Answer from the drawing. Dimensions are ordinates in mm from the lowest x, y and z of the part. A direction names the side the tool comes from. Round coordinates to 2 decimals unless told otherwise and drop trailing zeros. Loops run counter-clockwise (first coordinate to the right, second up) from the corner with the lowest first, then second, coordinate; pieces in that order, holes last. Notation, with made-up numbers: M -3.75,59.25 L 9.25,59.25 A24 ccw 9.25,87.25 Z; hole C 3.25,14 d3. An arc over 180 degrees is marked long. One line per item, written item: value.
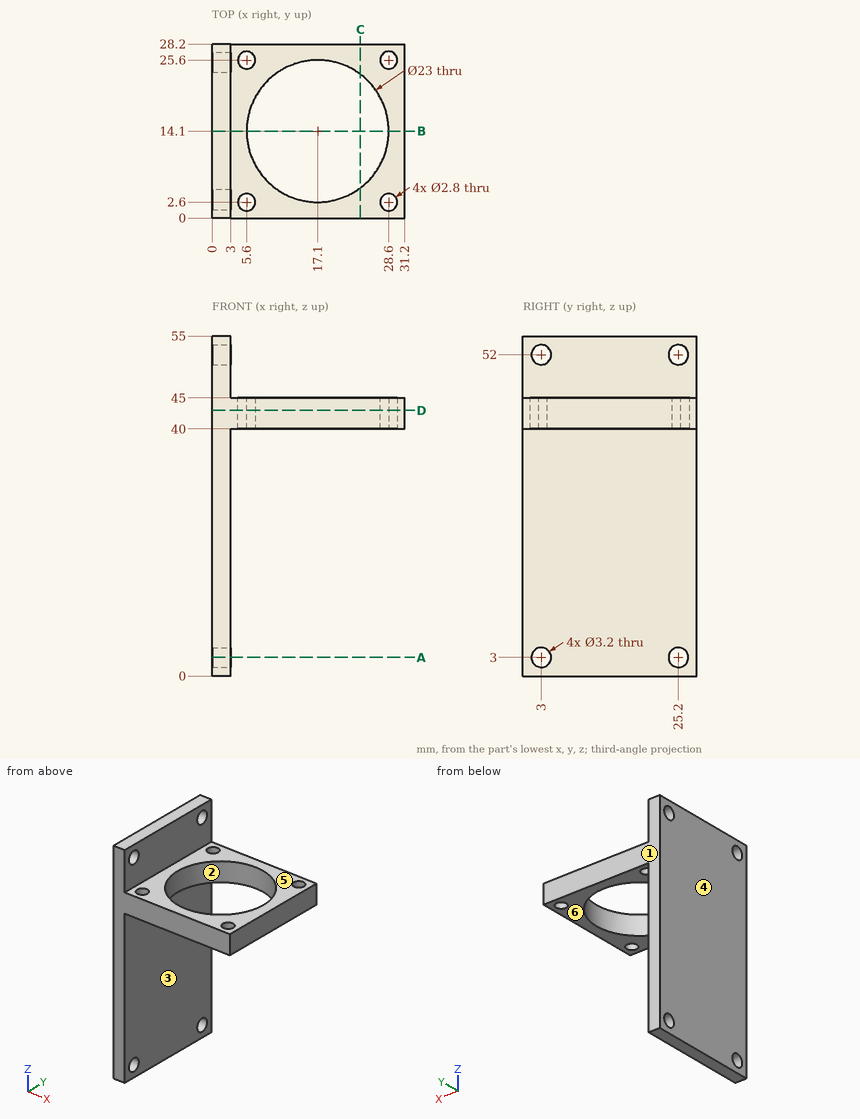
1) Find section C-C (x = 24). Give the vertices of the cut face in (y, z).
Check values:
outline: M 0,40 L 4.9,40 L 4.9,45 L 0,45 Z; M 23.3,40 L 28.2,40 L 28.2,45 L 23.3,45 Z
2) Find the intervals of material crossed by probe 1 along Z at (x, y) = (1.45, 25.2); probe 2 along X at (y, z) = (26.5, 24.5); probe 3 along Z at (x, y) = (29.5, 15.5), in increasing order. Write a range as from..to.
Check values:
probe 1: 0..1.4, 4.6..50.4, 53.6..55
probe 2: 0..3
probe 3: 40..45
3) Each of these flat-tipped pins is pushed along its axis until it touches: pin 1 (1.7 mm diameter, centred on x = 28.6, y = 25.6, fed in from +Z); pin 2 (3 mm diameter, centred on y = 11.5, z = 49, fed in from +X); pin 3 (4.5 mm diameter, centred on x = 5.6, y = 2.6, fed in from +Z); pin 4 (10 mm diameter, centred on x = 23, z = 46, fed in from +Y). Where does it stop, or does it pass through?
Check values:
pin 1: through
pin 2: x = 3
pin 3: z = 45
pin 4: y = 28.2
4) The mould has two halves that part along X. Classify the marked faces 1, 2 and 3: +X half, -X half, draft (parallel to the pull), parting line (faces both ways), or undercut.
Check values:
face 1: draft
face 2: undercut
face 3: +X half
5) Find section B-B (y = 14.1). Give the vertices of the cut face in (x, z).
Check values:
outline: M 0,0 L 3,0 L 3,40 L 5.6,40 L 5.6,45 L 3,45 L 3,55 L 0,55 Z; M 28.6,40 L 31.2,40 L 31.2,45 L 28.6,45 Z
6) For the marked faces 4, 5 and 6, determine the directions among +Z, -Z, +X, -X, +Y, -Y from which every point of the face is accessible in a straight line to the end or side of a thin tool.
Check values:
face 4: +Z, -Z, -X, +Y, -Y
face 5: +Z, +X, +Y, -Y
face 6: -Z, +X, +Y, -Y
7) Find section A-A (z = 3). Give the vertices of the cut face in (x, y).
Check values:
outline: M 0,0 L 3,0 L 3,1.4 L 0,1.4 Z; M 0,4.6 L 3,4.6 L 3,23.6 L 0,23.6 Z; M 0,26.8 L 3,26.8 L 3,28.2 L 0,28.2 Z
8) Find section D-D (z = 43). Give the vertices of the cut face in (x, y), then the cut area to 3 significant figures.
Check values:
outline: M 0,0 L 31.2,0 L 31.2,28.2 L 0,28.2 Z; hole C 5.6,2.6 d2.8; hole C 5.6,25.6 d2.8; hole C 17.1,14.1 d23; hole C 28.6,2.6 d2.8; hole C 28.6,25.6 d2.8
area: 440 mm2
